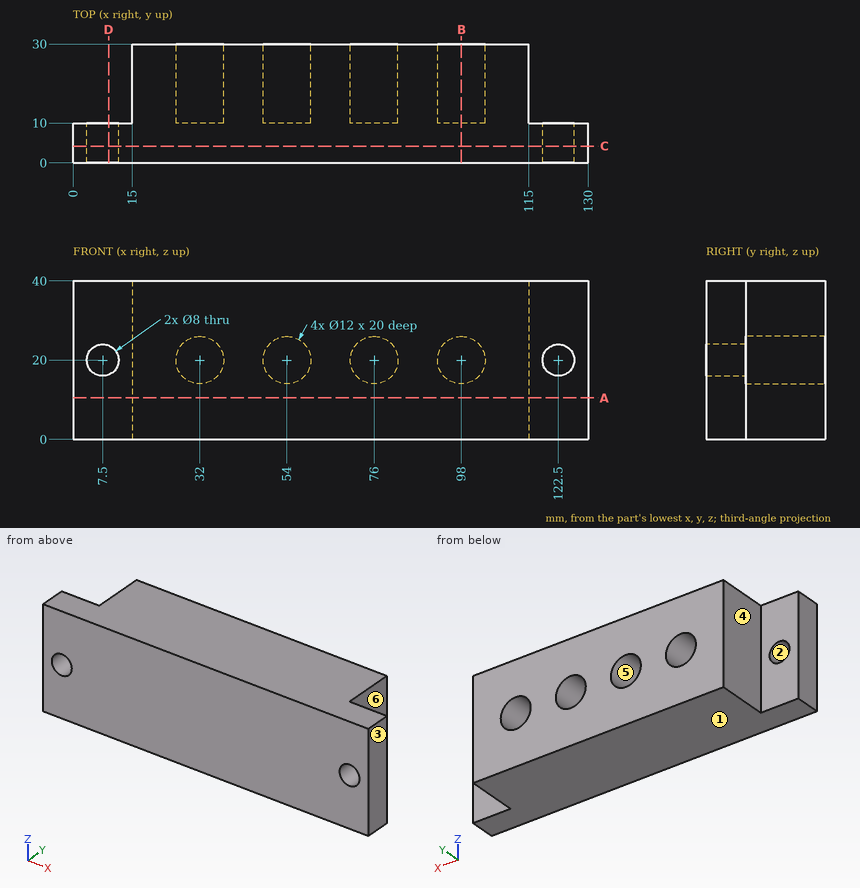
The drawing under review shows one solid part. Ordinate dimensions are in mm from its lowest x, y, z. A direction names the side the tool comes from. Round coordinates to 2 decimals unless told otherwise and drop trailing zeros. Loops run counter-clockwise (first coordinate to the right, second up) from the corner with the lowest first, then second, coordinate; pieces in that order, holes last. Notation, with made-up numbers: (53.5, -2) - (108.5, -2) arc R17 ccw to (108.5, 17) - close; hole circle Ø1 at (18.5, 27.5). An arc over 180 degrees is marked (long way). Use a Markdown table: item, result. Add a question column.
Q1. Add section B-B (x = 98). State the section outline as (y, z) points, plus the area to 3 significant figures.
Q2. Machinability: for the marked faces 4, 5 and 6, which of the approach directions +Z, -Z, +X, -X, +Y, -Y give a long, thin tool a straight path to every point of the face, cutting with its end or side? Answer none if there is none.
Q3. Add section D-D (x = 9). State the section outline as (y, z) points, plus the area to 3 significant figures.
Q4. For probe 1 along X at (y, z) = (20.5, 20); probe 2 along X at (y, z) = (6.25, 20); probe 3 along Z at (x, y) = (75.5, 11.25), list the stretches that pass through material, from the lowest coordinate up.
Q5. Add section C-C (y = 4.25). State the section outline as (x, z) points, plus the area to 3 significant figures.
Q6. The part is to be moulded in two halves that separate along Z. For the marked faces 1, 2 and 3, say which applies: pulls with the +Z half, pulls with the -Z half, needs draft (parallel to the pull), parting line crosses it, or undercut.
Q7. Insertion check: pin 1 Ø13 at (x, z) = (7.5, 20) entering from +Y; pin 2 Ø5 at (x, z) = (28.5, 18.5) entering from -Y; pin 3 Ø16 at (y, z) = (21.5, 26) entering from +X; pin 4 Ø6 at (y, z) = (18, 14.5) entering from -X. Each pin has a flat end and moves straight along its axis. Give the tip position at first contact, or say it passes through.
Q8. Add section A-A (z = 10.5). State the section outline as (x, y) points, plus the area to 3 significant figures.
Worked answers:
| question | item | result |
|---|---|---|
| 1 | outline | (0, 0) - (30, 0) - (30, 14) - (10, 14) - (10, 26) - (30, 26) - (30, 40) - (0, 40) - close |
| 1 | area | 960 mm² |
| 2 | face 4 | +Z, -Z, -X, +Y |
| 2 | face 5 | +Y |
| 2 | face 6 | +Z, -Z, +X, +Y |
| 3 | outline | (0, 0) - (10, 0) - (10, 16.29) - (0, 16.29) - close; (0, 23.71) - (10, 23.71) - (10, 40) - (0, 40) - close |
| 3 | area | 326 mm² |
| 4 | probe 1 | 15 to 26, 38 to 48, 60 to 70, 82 to 92, 104 to 115 |
| 4 | probe 2 | 0 to 3.5, 11.5 to 118.5, 126.5 to 130 |
| 4 | probe 3 | 0 to 14.02, 25.98 to 40 |
| 5 | outline | (0, 0) - (130, 0) - (130, 40) - (0, 40) - close; hole circle Ø8 at (7.5, 20); hole circle Ø8 at (122.5, 20) |
| 5 | area | 5,100 mm² |
| 6 | face 1 | pulls with the -Z half |
| 6 | face 2 | undercut |
| 6 | face 3 | needs draft |
| 7 | pin 1 | y = 10 |
| 7 | pin 2 | y = 0 |
| 7 | pin 3 | x = 115 |
| 7 | pin 4 | x = 15 |
| 8 | outline | (0, 0) - (130, 0) - (130, 10) - (115, 10) - (115, 30) - (15, 30) - (15, 10) - (0, 10) - close |
| 8 | area | 3,300 mm² |
